Could you check a few things on this drawing? It's one solid part, dimensions in mm from its lowest x, y, z. Give positions to 0.01 mm unless a question says otherwise; leave off trailing zeros. Loops run counter-clockwise (first coordinate to the right, second up) from the corner with the lowest first, then second, coordinate; pieces in that order, holes last. Notation, with made-up numbers: M -37,-20 L -9,-20 A29 ccw -9,15 Z; hole C -9,33.25 d10. An arc over 180 degrees is marked long. Answer as a JSON object with one key per item and string values.
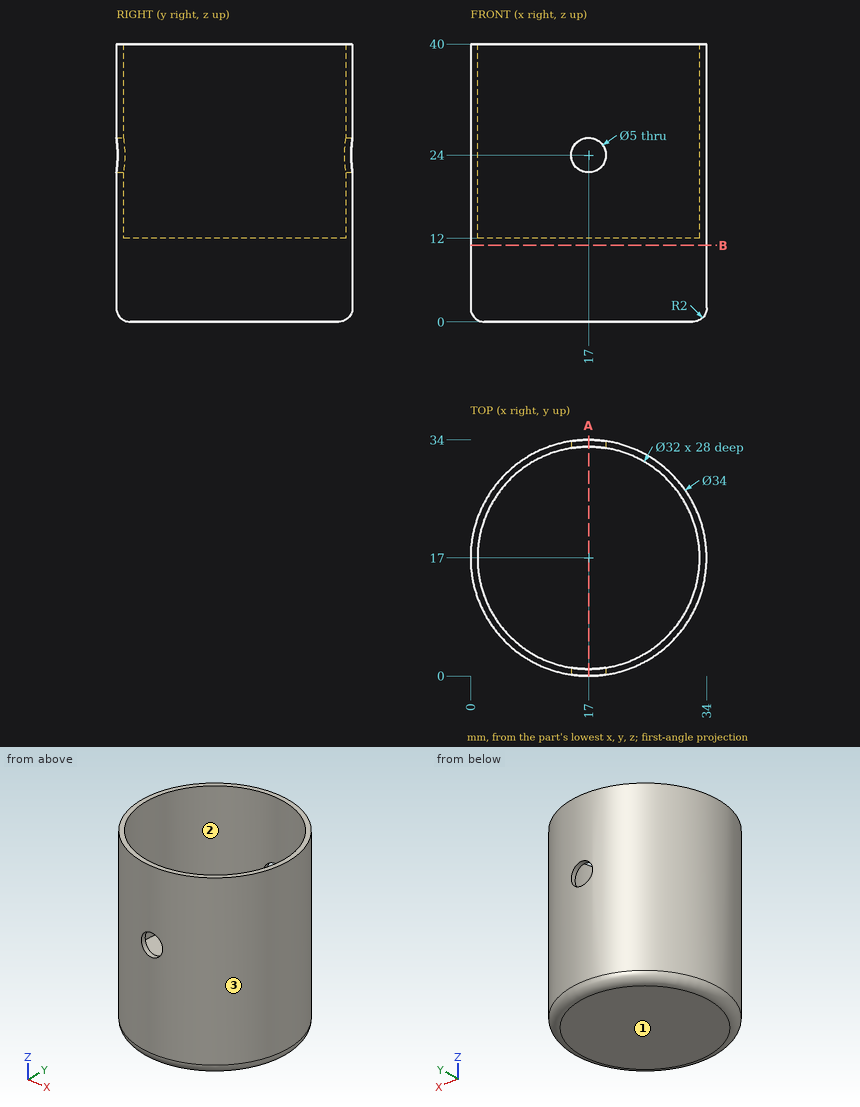
1) Please list where these lines run through material, in increasing order: line 1 along Z through (x, y) = (26.5, 16.5); line 2 along X through (y, z) = (25, 11.5); line 3 along Y through (x, z) = (16.5, 20). Write a range as from..to.
Answer list:
{"line 1": "0..12", "line 2": "2..32", "line 3": "0.01..1.01, 32.99..33.99"}
2) Will these pins go through, and if not, where does the flat tip stop? pin 1 Ø1.5 at (y, z) = (15.5, 35) entering from +X; pin 2 Ø10 at (x, y) = (25.5, 13.5) entering from +Z; pin 3 Ø6 at (y, z) = (10, 9.5) entering from -X.
Answer list:
{"pin 1": "x = 33.98", "pin 2": "z = 12", "pin 3": "x = 0.48"}
3) Suppose I cut it at A-A, the plane x = 17. Give the number of separate pieces and of enclosed holes in the cut face, and give its area (3 significant figures).
Answer list:
{"separate pieces": "3", "enclosed holes": "0", "area": "452 mm^2"}
4) Suppose I cut it at B-B, the plane z = 11. Write out the boundary of the cut face in (x, y), and give its area (3 significant figures).
Answer list:
{"outline": "C 17,17 d34", "area": "908 mm^2"}
5) If we mould it in two halves opening along Y, with no side actions, what happens to the marked faces 1, 2 and 3? For each: +Y half, -Y half, draft (parallel to the pull), parting line (faces both ways), or undercut.
Answer list:
{"face 1": "draft", "face 2": "undercut", "face 3": "parting line"}
